```python
from build123d import *

# Parameters (mm, degrees)
F0_W    = 15.0114
F0_H    = 17.4625
F0_W_2  = 7.2136
F0_H_2  = 10.287
F2_R    = 1.5875
F3_SIZE = 0.79375


# Not quite as in the source:
# - a fillet or chamfer that OpenCascade refuses, or shapes differently, is made with other operations: its cross-section is extruded or revolved along the edge and cut away or added


with BuildPart() as f1:
    # F0 (on Right) → F1 (revolve)
    with BuildSketch(Plane.YZ):
        with Locations((14.7193, 16.66875)):
            Rectangle(F0_W, F0_H)
        with Locations((3.6068, 16.66875)):
            Rectangle(F0_W_2, F0_H)
        with Locations((3.6068, 30.5435)):
            Rectangle(F0_W_2, F0_H_2)
    revolve(axis=Axis((0, 11.1125, 0), (0, 1, 0)))

    # F2
    f2_edges = [f1.edges().sort_by_distance(p)[0] for p in [
        (0, 7.2136, -25.4),
    ]]
    fillet(f2_edges, radius=F2_R)

    # F3
    f3_edges = [f1.edges().sort_by_distance(p)[0] for p in [
        (0, 22.225, -25.4),
    ]]
    chamfer(f3_edges, length=F3_SIZE)

    # F4: chamfer of 6.35 x 15.748 on 2 edges, made by hand

    # F4_s1 → F4_t2 (revolve, cut)
    with BuildSketch(Plane.YZ):
        Polygon((15.748, 35.687), (0, 29.337), (0, 35.687), align=None)
    revolve(axis=Axis((0, 0, 0), (0, 1, 0)), mode=Mode.SUBTRACT)


solid = f1.part
```
Geometry check sheet. Reference: the model listing, model coordinates, mm. A direction names the side the tool comes from. Give positions to 0.01 mm unless a question says otherwise; leave off trailing zeros. Loops run counter-clockwise (first coordinate to the right, second up) from the corner with the lowest first, then second, coordinate; pieces in that order, holes last. Notation, with made-up numbers: M 67.5,2.5 L 71.5,2.5 A16 ccw 71.5,19.5 Z; hole C -40,67.5 d1. An arc over 180 degrees is marked long. Write item = value, one per line.
(1) Sectioned sample at C-C, the plane y = 16. Record the cut outline in (x, z) (1 decimal).
Answer below:
outline = C 0,0 d50.8; hole C 0,0 d15.9
(2) Sectioned sample at D-D, the plane y = 4.5. Record the cut outline in (x, z) (1 decimal).
Answer below:
outline = C 0,0 d62.3; hole C 0,0 d15.9
(3) Material ranges on line 1 (X direction, y = 16.5, z = 0); line 2 (X direction, y = 19, z = 6); line 3 (Z direction, x = 7, y = 16), recorded low to high. Write a range as [from, to].
Answer below:
line_1 = [-25.4, -7.94], [7.94, 25.4]
line_2 = [-24.68, -5.2], [5.2, 24.68]
line_3 = [-24.42, -3.74], [3.74, 24.42]
(4) Tool access check on faces 1 (the face through (-21.3, 7.214, 16.9)), 2 (the face through (-6, 0, 6)). Record the directions out of +Z, -Z, +X, -X, +Y, -Y that give a thin tool (end or side, any length) a straight path to the whole face; none if there is none.
Answer below:
face_1 = +Y
face_2 = +Z, -Z, +X, -X, -Y
(5) Sectioned sample at A-A, the plane x = 0. Record the cut outline in (y, z) (1 decimal).
Answer below:
outline = M 0,-29.3 L 7.2,-32.2 L 7.2,-27 A1.6 cw 8.8,-25.4 L 21.4,-25.4 L 22.2,-24.6 L 22.2,-7.9 L 0,-7.9 Z; M 0,7.9 L 22.2,7.9 L 22.2,24.6 L 21.4,25.4 L 8.8,25.4 A1.6 cw 7.2,27 L 7.2,32.2 L 0,29.3 Z
(6) Sectioned sample at B-B, the plane z = 0. Record the cut outline in (x, y) (1 decimal), plus the area to 3 significant figures.
Answer below:
outline = M -32.2,7.2 L -29.3,0 L -7.9,0 L -7.9,22.2 L -24.6,22.2 L -25.4,21.4 L -25.4,8.8 A1.6 cw -27,7.2 Z; M 7.9,0 L 29.3,0 L 32.2,7.2 L 27,7.2 A1.6 cw 25.4,8.8 L 25.4,21.4 L 24.6,22.2 L 7.9,22.2 Z
area = 854 mm2
(7) Release check for a two-part mould opening along X. For faces 3 (the face through (-24.796, 15.028, -5.506)), 4 (the face through (6, 22.225, 6)), 5 (the face through (-7.75, 11.27, -1.72)) record: released by +X, released by -X, zero draft, split by the parting line, or undercut.
Answer below:
face_3 = split by the parting line
face_4 = zero draft
face_5 = undercut
(8) Gauge pin test, flat ends, axial feed: pin 1 Ø5 at (y, z) = (16.5, -16.5) entering from +X; pin 2 Ø6 at (x, y) = (16, 19) entering from -Z; pin 3 Ø1 at (y, z) = (18.5, 9.5) entering from +X. Record the tip position at first contact, or that the pin passes through.
Answer below:
pin_1 = 21.19
pin_2 = -21.82
pin_3 = 23.75
